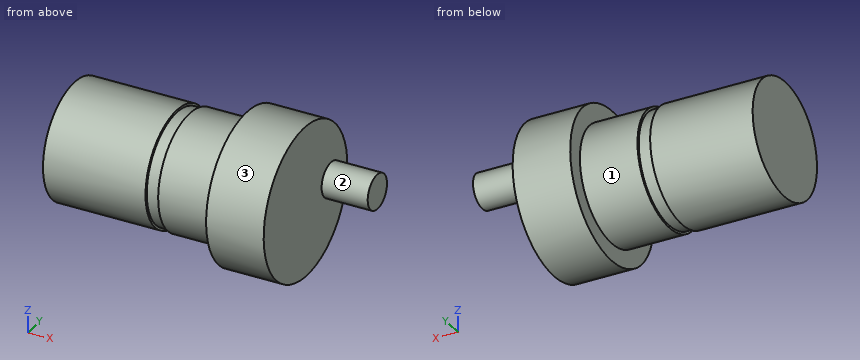
from build123d import *

# Parameters (mm, degrees)
SKETCH1_R           = 6.5
BOSS_EXTRUDE1_DEPTH = 5
SKETCH2_R           = 5
BOSS_EXTRUDE2_DEPTH = 15
SKETCH3_R           = 1.5
BOSS_EXTRUDE3_DEPTH = 4
SKETCH4_W           = 1.1
SKETCH4_H           = 0.2


with BuildPart() as part:
    # Sketch1 → Boss-Extrude1 (new body)
    with BuildSketch(Plane(origin=(0, 0, 0), x_dir=(0, 0, -1), z_dir=(1, 0, 0))):
        Circle(SKETCH1_R)
    extrude(amount=BOSS_EXTRUDE1_DEPTH)

    # Sketch2 → Boss-Extrude2 (add)
    with BuildSketch(Plane.ZY):
        Circle(SKETCH2_R)
    extrude(amount=BOSS_EXTRUDE2_DEPTH)

    # Sketch3 → Boss-Extrude3 (add)
    with BuildSketch(Plane(origin=(5, 0, 0), x_dir=(0, 0, -1), z_dir=(1, 0, 0))):
        with Locations((0, 4)):
            Circle(SKETCH3_R)
    extrude(amount=BOSS_EXTRUDE3_DEPTH)

    # Sketch4 → Cut-Revolve1 (revolve, cut)
    with BuildSketch(Plane.XY):
        with Locations((-5.55, 4.9)):
            Rectangle(SKETCH4_W, SKETCH4_H)
    revolve(axis=Axis((-1.178470482, 0, 0), (-1, 0, 0)), mode=Mode.SUBTRACT)


solid = part.part
Check sheet for the modelled part. Datum: model origin and axes. Units: mm. Face numbers are marked on the shaded views. A direction names the side the tool comes from. Coordinates: 2 decimals unless noted, no trailing zeros. Write each loop counter-clockwise with the first axis right and the second up, starting at its lowest first coordinate (ties: lowest second). Pieces come first, ordered by that corner, then holes. Notation, with made-up numbers: M 50,35.25 L 78,35.25 A20 cw 78,53.25 Z; hole C -24,77.25 d10. An arc over 180 degrees is marked long. Answer as CSV lines item,"result".
Q1. Cross-section at B-B (z = 0). Record the boundary of the cut face in (x, y), then the cut area to 3 significant figures.
Check result:
outline,"M -15,-5 L -6.1,-5 L -6.1,-4.8 L -5,-4.8 L -5,-5 L 0,-5 L 0,-6.5 L 5,-6.5 L 5,2.5 L 9,2.5 L 9,5.5 L 5,5.5 L 5,6.5 L 0,6.5 L 0,5 L -5,5 L -5,4.8 L -6.1,4.8 L -6.1,5 L -15,5 Z"
area,"227 mm^2"
Q2. Material ranges on probe 1 along X at (y, z) = (-5, -1.5); probe 2 along X at (y, z) = (-2.5, -2.5); probe 3 along Z at (x, y) = (-0.25, 1.75), recorded low to high. Write a range as from..to.
Check result:
probe 1,"0..5"
probe 2,"-15..5"
probe 3,"-4.68..4.68"
Q3. Set-up check for the marked faces 1, 2 and 3: record each of +Z, -Z, +X, -X, +Y, -Y from which the full face is reachable in a straight line by a thin tool's end or side.
Check result:
face 1,"-X"
face 2,"+X"
face 3,"+X, -X"
Q4. Cross-section at C-C (x = 1.5). Record the boundary of the cut face in (y, z), then the cut area to 3 significant figures.
Check result:
outline,"C 0,0 d13"
area,"133 mm^2"
Q5. Go/stop test with flat-tipped pins: pin 1 (4 mm diameter, centred on x = -7.5, y = 0.5, fed in from +Z); pin 2 (1.5 mm diameter, centred on x = -8, y = -1, fed in from -Z); pin 3 (4 mm diameter, centred on x = 1, z = -2.5, fed in from -Y). Record where each tip stops, or that it passes through.
Check result:
pin 1,"z = 5"
pin 2,"z = -4.99"
pin 3,"y = -6.48"
Q6. Cross-section at D-D (z = -4.5). Record the boundary of the cut face in (x, y), then the cut area to 3 significant figures.
Check result:
outline,"M -15,-2.18 L -6.1,-2.18 L -6.1,-1.67 L -5,-1.67 L -5,-2.18 L 0,-2.18 L 0,-4.69 L 5,-4.69 L 5,4.69 L 0,4.69 L 0,2.18 L -5,2.18 L -5,1.67 L -6.1,1.67 L -6.1,2.18 L -15,2.18 Z"
area,"111 mm^2"
Q7. Cross-section at A-A (y = 0). Record the boundary of the cut face in (x, z).
Check result:
outline,"M -15,-5 L -6.1,-5 L -6.1,-4.8 L -5,-4.8 L -5,-5 L 0,-5 L 0,-6.5 L 5,-6.5 L 5,6.5 L 0,6.5 L 0,5 L -5,5 L -5,4.8 L -6.1,4.8 L -6.1,5 L -15,5 Z"
